Can you work these out from the model? Positions are in its coordinate system, mm. Face numbers are marked on the shaded views. A direction names the side the tool comes from. Round coordinates to 2 decimals unless told otherwise and drop trailing zeros. Loops run counter-clockwise (first coordinate to the right, second up) from the corner with the lowest first, then second, coordinate; pieces in that order, holes last. Notation, with made-up numbers: M -31.5,-9 L -14.5,-9 A17 ccw -14.5,14 Z; hole C 38.25,86.25 d5. An arc over 180 degrees is marked long. Answer as CSV lines item,"result".
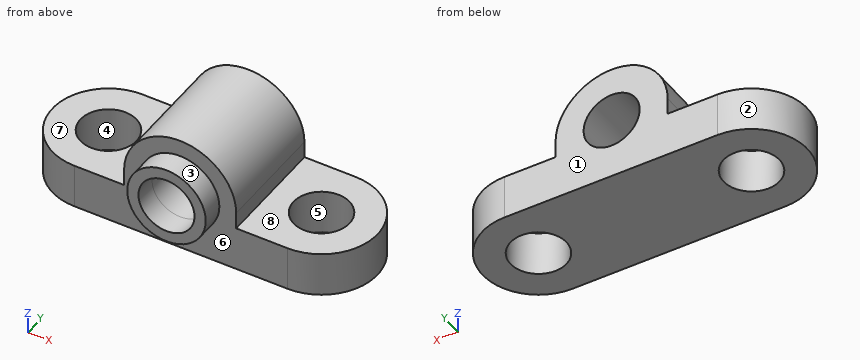
from build123d import *

# Parameters (mm, degrees)
F0_R     = 5
F1_DEPTH = 8
F3_DEPTH = 20
F4_R     = 5
F5_DEPTH = 20.001
F4_R_2   = 7
F6_DEPTH = 4


with BuildPart() as f1:
    # F0 (on Top) → F1 (new body)
    with BuildSketch(Plane.XY):
        with BuildLine():
            ThreePointArc((-18.86745, 8.988079), (-28.86745, -1.011921), (-18.86745, -11.011921))
            Line((-18.86745, -11.011921), (19.13255, -11.011921))
            ThreePointArc((19.13255, -11.011921), (29.13255, -1.011921), (19.13255, 8.988079))
            Line((19.13255, 8.988079), (-18.86745, 8.988079))
        make_face()
        with Locations((-18.86745, -1.011921)):
            Circle(F0_R, mode=Mode.SUBTRACT)
        with Locations((19.13255, -1.011921)):
            Circle(F0_R, mode=Mode.SUBTRACT)
    extrude(amount=F1_DEPTH)

    # F2 (on face) → F3 (join)
    with BuildSketch(Plane.XZ.offset(11.011921)):
        Polygon((-10, 11), (-10, 8), (0, 8), (10, 8), (10, 11), (0, 11), align=None)
        with BuildLine():
            ThreePointArc((10, 11), (0, 21), (-10, 11))
            Line((-10, 11), (0, 11))
            Line((0, 11), (10, 11))
        make_face()
    extrude(amount=-F3_DEPTH)

    # F4 (on face) → F5 (cut, through all)
    with BuildSketch(Plane.XZ.offset(11.011921)):
        with Locations((0, 11)):
            Circle(F4_R)
    extrude(amount=-F5_DEPTH, mode=Mode.SUBTRACT)

    # F4 (on face) → F6 (join)
    with BuildSketch(Plane.XZ.offset(11.011921)):
        with Locations((0, 11)):
            Circle(F4_R_2)
        with Locations((0, 11)):
            Circle(F4_R, mode=Mode.SUBTRACT)
    extrude(amount=F6_DEPTH)


solid = f1.part
Item 1: If we section it at B-B on x = 0: Write out the boundary of the cut face in (y, z), then the cut area to 3 significant figures.
Output:
outline,"M -15.01,4 L -11.01,4 L -11.01,0 L 8.99,0 L 8.99,6 L -15.01,6 Z; M -15.01,16 L 8.99,16 L 8.99,21 L -11.01,21 L -11.01,18 L -15.01,18 Z"
area,"236 mm2"
Item 2: If I drill on line 1 along X through (y, z) = (-0.25, 3.5); line 2 along Z through (x, y) = (0, -12.3); line 3 along Y through (x, z) = (-9, 2.5), over which ranges is the centre line in solid material (lowest first)? Write a range as from..to.
Output:
line 1,"x = -28.84..-23.81, -13.93..14.19, 24.07..29.1"
line 2,"z = 4..6, 16..18"
line 3,"y = -11.01..8.99"
Item 3: If we section it at C-C on z = 6.75: Write out the boundary of the cut face in (x, y).
Output:
outline,"M -18.87,-11.01 L -5.56,-11.01 L -5.56,-15.01 L -2.63,-15.01 L -2.63,8.99 L -18.87,8.99 A10 ccw Z; M 2.63,-15.01 L 5.56,-15.01 L 5.56,-11.01 L 19.13,-11.01 A10 ccw 19.13,8.99 L 2.63,8.99 Z; hole C -18.87,-1.01 d10; hole C 19.13,-1.01 d10"
Item 4: Will these pins go through, and if not, where does the flat tip stop? pin 1 (9.5 mm diameter, centred on x = -16, y = 1, fed in from +Z); pin 2 (2 mm diameter, centred on y = 1, z = 18.5, fed in from +X); pin 3 (2.5 mm diameter, centred on y = -4, z = 9.5, fed in from -X).
Output:
pin 1,"stops at z = 8"
pin 2,"stops at x = 7.6"
pin 3,"stops at x = -10"
Item 5: On a 3-axis mill with a long thin cutter (end or side, diameter ignored), from which of +Z, -Z, +X, -X, +Y, -Y can I reach the whole of each face in a straight line? I mean the marked faces 5, 6, 7 and 8. Say none if no direction works.
Output:
face 5,"+Z, -Z"
face 6,"-Y"
face 7,"+Z, -X, +Y, -Y"
face 8,"+Z, +X, +Y, -Y"
Item 6: We'd pull the mould along X, two halves only. Please class the marked faces 1, 2, 3 and 4: released by +X, released by -X, zero draft, split by the parting line, or undercut.
Output:
face 1,"zero draft"
face 2,"released by -X"
face 3,"split by the parting line"
face 4,"undercut"
Item 7: If we section it at A-A on y = -4.25: Write out the boundary of the cut face in (x, z).
Output:
outline,"M -28.33,0 L -22.68,0 L -22.68,8 L -28.33,8 Z; M -15.06,0 L 15.32,0 L 15.32,8 L 10,8 L 10,11 A10 ccw -10,11 L -10,8 L -15.06,8 Z; M 22.94,0 L 28.59,0 L 28.59,8 L 22.94,8 Z; hole C 0,11 d10"
Item 8: If we section it at D-D on y = -9.25: Write out the boundary of the cut face in (x, z).
Output:
outline,"M -24.54,0 L 24.8,0 L 24.8,8 L 10,8 L 10,11 A10 ccw -10,11 L -10,8 L -24.54,8 Z; hole C 0,11 d10"
